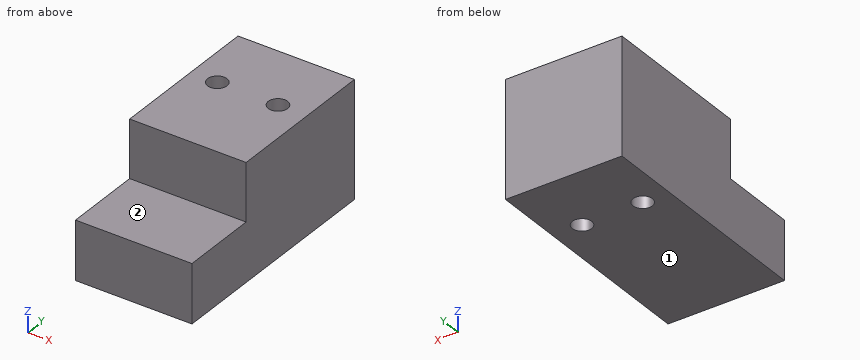
from build123d import *

# Parameters (mm, degrees)
F0_W     = 76.2
F0_H     = 152.4
F1_DEPTH = 76.2
F2_R     = 6.35
F3_DEPTH = 76.2
F4_W     = 76.2
F4_H     = 38.1
F5_DEPTH = 25.4
F6_DEPTH = 50.8


with BuildPart() as f1:
    # F0 (on Top) → F1 (new body)
    with BuildSketch(Plane.XY):
        with Locations((16.290675, -17.46637)):
            Rectangle(F0_W, F0_H)
    extrude(amount=F1_DEPTH)

    # F2 (on face) → F3 (cut)
    with BuildSketch(Plane.XY.offset(76.2)):
        with Locations((-4.356702, 14.28363)):
            Circle(F2_R)
        with Locations((35.340675, 14.28363)):
            Circle(F2_R)
    extrude(amount=-F3_DEPTH, mode=Mode.SUBTRACT)

    # F4 (on face) → F5 (cut)
    with BuildSketch(Plane.XZ.offset(93.66637)):
        with Locations((16.290675, 57.446664)):
            Rectangle(F4_W, F4_H)
    extrude(amount=-F5_DEPTH, mode=Mode.SUBTRACT)

    # F4 (on face) → F6 (cut)
    with BuildSketch(Plane.XZ.offset(93.66637)):
        with Locations((16.290675, 57.446664)):
            Rectangle(F4_W, F4_H)
    extrude(amount=-F6_DEPTH, mode=Mode.SUBTRACT)


solid = f1.part
Here's how the part is built. I have some questions about the finished solid (model axes, mm). Face numbers are marked on the shaded views. A direction names the side the tool comes from. Coordinates: 2 decimals unless noted, no trailing zeros. Order: outer loops, then holes, each group sorted by start corner. A loop starts at its lowest first (then second) coordinate and runs counter-clockwise, first axis right, second up.
Item 1: If we section it at A-A on x = 31.5: List the corners of the cut face in (y, z) for me.
Result sheet:
outline: (-93.67, 0) - (9.23, 0) - (9.23, 76.2) - (-42.87, 76.2) - (-42.87, 38.4) - (-93.67, 38.4) - close; (19.34, 0) - (58.73, 0) - (58.73, 76.2) - (19.34, 76.2) - close
Item 2: For the marked faces 1 and 2, which set-ups out of +Z, -Z, +X, -X, +Y, -Y let a thin tool reach every point of the face, with its end or its side?
Result sheet:
face 1: -Z, +X, -X, +Y, -Y
face 2: +Z, +X, -X, -Y
Item 3: If we section it at B-B on z = 25.5: List the corners of the cut face in (x, y) for me.
Result sheet:
outline: (-21.81, -93.67) - (54.39, -93.67) - (54.39, 58.73) - (-21.81, 58.73) - close; hole circle Ø12.7 at (-4.36, 14.28); hole circle Ø12.7 at (35.34, 14.28)
Item 4: For P1, Ø11.5, axis at x = -4.36, y = 14.28, coming from the -Z side; P2, Ø19, axis at x = 11, z = 58, coming from the -Y side; P3, Ø15, axis at x = 22.5, y = -68.5, coming from the +Z side, each with a flat end and sliding along its axis, tell me the tip position at first contact or that it passes through.
Result sheet:
P1: passes through
P2: stops at y = -42.87
P3: stops at z = 38.4
Item 5: If we section it at C-C on y = -53.5: List the corners of the cut face in (x, z) for me.
Result sheet:
outline: (-21.81, 0) - (54.39, 0) - (54.39, 38.4) - (-21.81, 38.4) - close
Item 6: If we section it at D-D on x = -3: List the corners of the cut face in (y, z) for me.
Result sheet:
outline: (-93.67, 0) - (8.08, 0) - (8.08, 76.2) - (-42.87, 76.2) - (-42.87, 38.4) - (-93.67, 38.4) - close; (20.49, 0) - (58.73, 0) - (58.73, 76.2) - (20.49, 76.2) - close
Item 7: I need wall thicknesses on line 1 (X direction, y = 12, z = 71); line 2 (Y direction, x = 25, z = 59); line 3 (Z direction, x = 14.5, y = -73). Which ranges of each line are inside material? Lowest first, please.
Result sheet:
line 1: x = -21.81 to -10.28, 1.57 to 29.42, 41.27 to 54.39
line 2: y = -42.87 to 58.73
line 3: z = 0 to 38.4
